Part model, mm, in its own coordinate system. A direction names the side the tool comes from. Round coordinates to 2 decimals unless told otherwise and drop trailing zeros. Loops run counter-clockwise (first coordinate to the right, second up) from the corner with the lowest first, then second, coordinate; pieces in that order, holes last. Notation, with made-up numbers: (42.5, 38) -> (95.5, 38) arc R26 ccw to (95.5, 69) -> close; hole circle Ø11 at (68.25, 20.5). An arc over 180 degrees is marked (long way). Use a Markdown table: item, result. Add a question column.
Item 1: Probe line 1 (Z direction, x = -113, y = 4.5) (3 decimals); line 2 (X direction, y = 73, z = 21.5); line 3 (Y direction, x = -144.5, z = 103.5). List the from-to ranges inside material, lowest first. Write a range as [from, to].
Item 2: Cut at A-A, the plane z = 20. List the corners of the cut face in (x, y), plus the area to 3 significant figures.
Item 3: Cut at B-B, the plane x = -57. List the corners of the cut face in (y, z) (3 decimals), plus the area to 3 significant figures.
Item 4: Flat gauge pins, fed straight in: pin 1 (1 mm diameter, centred on y = -4.5, z = 16.5, fed in from -X); pin 2 (10 mm diameter, centred on y = 34, z = 69, fed in from -X); pin 3 (1.5 mm diameter, centred on x = -155.5, z = 60, fed in from -Y). Where does each tip first touch, or does it go through?
Item 5: Cut at C-C, the plane y = 70. List the corners of the cut face in (x, z) (3 decimals).
Item 6: Which spindle directions (+Z, -Z, +X, -X, +Y, -Y) get a long thin tool onto all of the face, cutting with end or side? Do faces 1 (the face through (-43.02, 64.44, 62.61)), 2 (the face through (-92.102, 86.004, 67.44)). Say none if no direction does.
```python
from build123d import *

# Parameters (mm, degrees)
F1_DEPTH = 127
F2_T     = -9.525


# Not quite as in the source:
# - a length typed as a fraction of an inch, garbled in the dataset ("3 / 203.2 mm" for 3/8 in), is restored


with BuildPart() as f1:
    # F0 (on Top) → F1 (new body)
    with BuildSketch(Plane.XY):
        Polygon((-25.8614264401, 39.6310188183), (-60.6637008516, 89.9540535799), (-120.8563842186, 100.9288884727), (-171.1794189802, 66.1266140612), (-182.154253873, 5.9339306942), (-147.3519794615, -44.3891040675), (-87.1592960945, -55.3639389602), (-36.8362613329, -20.5616645487), align=None)
    extrude(amount=F1_DEPTH)

    # F2
    f2_openings = [f1.faces().sort_by_distance(p)[0] for p in [
        (-104.00784, 22.782475, 127),
    ]]
    offset(amount=F2_T, openings=f2_openings)


solid = f1.part
```
A:
| question | item | result |
|---|---|---|
| 1 | line 1 | z = [0, 9.525] |
| 1 | line 2 | x = [-161.24, -144.5], [-60.52, -48.94] |
| 1 | line 3 | y = [-44.91, -31.77], [73, 84.58] |
| 2 | outline | (-182.15, 5.93) -> (-147.35, -44.39) -> (-87.16, -55.36) -> (-36.84, -20.56) -> (-25.86, 39.63) -> (-60.66, 89.95) -> (-120.86, 100.93) -> (-171.18, 66.13) -> close; hole (-172.08, 8.11) -> (-141.76, -35.73) -> (-89.33, -45.29) -> (-45.5, -14.97) -> (-35.94, 37.46) -> (-66.25, 81.29) -> (-118.68, 90.85) -> (-162.52, 60.54) -> close |
| 2 | area | 4,360 mm^2 |
| 3 | outline | (-34.506, 0) -> (84.656, 0) -> (84.656, 127) -> (67.911, 127) -> (67.911, 9.525) -> (-22.926, 9.525) -> (-22.926, 127) -> (-34.506, 127) -> close |
| 3 | area | 4,460 mm^2 |
| 4 | pin 1 | stops at x = -175.28 |
| 4 | pin 2 | stops at x = -177.95 |
| 4 | pin 3 | stops at y = -33.69 |
| 5 | outline | (-165.579, 0) -> (-46.864, 0) -> (-46.864, 127) -> (-58.445, 127) -> (-58.445, 9.525) -> (-148.833, 9.525) -> (-148.833, 127) -> (-165.579, 127) -> close |
| 6 | face 1 | +Z, -Z, +X, +Y |
| 6 | face 2 | +Z |
